Autodesk Inventor part; units mm, degrees
ref_plane "Work Plane1" through (-82.5, -59.605, 0) normal (0, 0, 1) x (1, 0, 0)
ref_plane "Work Plane2" through (-82.5, -59.605, 0) normal (0, 0, 1) x (1, 0, 0)
ref_plane "YZ Plane" through (0, 0, 0) normal (1, 0, 0) x (0, 1, 0)
ref_plane "Work Plane1" through (-82.5, -59.605, 0) normal (0, 0, 1) x (1, 0, 0)
sketch "Sketch1" plane through (0, 0, 0) normal (0, 0, 1) x (1, 0, 0)
  circle A0 centre (-78.95, -56.05) radius 1.75
  circle A1 centre (78.95, -56.05) radius 1.75
  circle A2 centre (78.95, 56.05) radius 1.75
  circle A3 centre (-78.95, 56.05) radius 1.75
  line L0 (-92.4724, 65.475) -> (91.6776, 65.475)
  line L1 (91.6776, 65.475) -> (91.6776, -64.7)
  line L2 (91.6776, -64.7) -> (-92.4724, -64.7)
  line L3 (-92.4724, -64.7) -> (-92.4724, 65.475)
  line L4 (-80.31, 46.61) -> (76.39, 46.61) construction
  line L5 (-80.31, -42.49) -> (-80.31, 46.61) construction
  line L6 (76.39, -42.49) -> (-80.31, -42.49) construction
  line L7 (76.39, 46.61) -> (76.39, -42.49) construction
  line L8 (-55.7212, -9.8482) -> (100.3438, -9.8482) construction
  line L9 (-82.2, -52) -> (82.2, -52) construction
  line L10 (-82.2, -52) -> (82.2, -52) construction
  circle A4 centre (-65.46, -58.76) radius 3.4
  circle A5 centre (-40.06, -58.76) radius 3.4
  circle A6 centre (-14.66, -58.76) radius 3.4
  circle A7 centre (10.74, -58.76) radius 3.4
  circle A8 centre (36.14, -58.76) radius 3.4
  circle A9 centre (61.54, -58.76) radius 3.4
  line L11 (82.5, -51.7) -> (82.5, 51.7)
  line L12 (82.2, 52) -> (-82.2, 52)
  line L13 (-82.5, 51.7) -> (-82.5, -51.7)
  line L14 (-82.2, -52) -> (82.2, -52)
  arc A10 (-82.2, 52) -> (-82.5, 51.7) centre (-82.2, 51.7) ccw
  arc A11 (82.5, 51.7) -> (82.2, 52) centre (82.2, 51.7) ccw
  arc A12 (82.2, -52) -> (82.5, -51.7) centre (82.2, -51.7) ccw
  arc A13 (-82.5, -51.7) -> (-82.2, -52) centre (-82.2, -51.7) ccw
  line L15 (-82.2, -53.27) -> (82.2, -53.27)
  arc A14 (82.2, -53.27) -> (83.77, -51.7) centre (82.2, -51.7) ccw
  line L16 (83.77, -51.7) -> (83.77, 51.7)
  arc A15 (83.77, 51.7) -> (82.2, 53.27) centre (82.2, 51.7) ccw
  line L17 (82.2, 53.27) -> (-82.2, 53.27)
  arc A16 (-82.2, 53.27) -> (-83.77, 51.7) centre (-82.2, 51.7) ccw
  line L18 (-83.77, 51.7) -> (-83.77, -51.7)
  arc A17 (-83.77, -51.7) -> (-82.2, -53.27) centre (-82.2, -51.7) ccw
  point P0 (-0.3974, -64.7)
  point P1 (-1.96, 65.475)
  dimension "d1" = 130.175
  dimension "d2" = 184.15
  dimension "d3" = 12.7
  dimension "d4" = 6.8
  dimension "d7" = 25.4
  dimension "d18" = 1.27
ref_plane "Work Plane2" through (-82.5, -59.605, 0) normal (0, 0, 1) x (1, 0, 0)
extrude "Extrusion2" add sketch "Sketch1" along normal blind 3.175 from surface at 0 contours L0 L1 L2 L3
properties part number "Center Bezel"
CAD build for the part. Positions are in the model's coordinates, mm. Coordinates: 2 decimals unless noted, no trailing zeros. Loops run counter-clockwise (first coordinate to the right, second up) from the corner with the lowest first, then second, coordinate; pieces in that order, holes last. Notation, with made-up numbers: (19.5, -24.75) - (59.5, -24.75) arc R16 ccw to (59.5, 1.25) - close; hole circle Ø11 at (34, 12.5). An arc over 180 degrees is marked (long way). Return JSON: item names as keys, results as strings.
1. Band-saw the part on B-B (x = -65.46). Give the cut face in (y, z) (3 decimals).
Result:
{"outline": "(-64.7, 0) - (-62.16, 0) - (-62.16, 3.175) - (-64.7, 3.175) - close; (-55.36, 0) - (-53.27, 0) - (-53.27, 3.175) - (-55.36, 3.175) - close; (53.27, 0) - (65.475, 0) - (65.475, 3.175) - (53.27, 3.175) - close"}
2. Drop a flat-ended pin along its axis: pin 1 (5.5 mm diameter, centred on x = 61.54, y = -58.76, fed in from +Z). Give the stop position or say it passes through.
Result:
{"pin 1": "passes through"}
3. Band-saw the part on A-A (y = -30.5). Give the cut face in (x, z) (3 decimals), and give its area (3 significant figures).
Result:
{"outline": "(-92.472, 0) - (-83.77, 0) - (-83.77, 3.175) - (-92.472, 3.175) - close; (83.77, 0) - (91.678, 0) - (91.678, 3.175) - (83.77, 3.175) - close", "area": "52.7 mm2"}
4. Band-saw the part on D-D (z = 1.9). State how many separate pieces and enclosed holes the cut face has, and give its area (3 significant figures).
Result:
{"separate pieces": "1", "enclosed holes": "11", "area": "5,870 mm2"}
5. Probe L1, parallel to Y at x = -40.06, z = 1.1 (3 decimals); L2, parallel to Y at x = 78.95, z = 1 (3 decimals); L3, parallel to X at y = -47, z = 1.25. List the from-to ranges inside material, lowest first. Write a range as from..to.
Result:
{"L1": "y = -64.7..-62.16, -55.36..-53.27, 53.27..65.475", "L2": "y = -64.7..-57.8, -54.3..-53.27, 53.27..54.3, 57.8..65.475", "L3": "x = -92.47..-83.77, 83.77..91.68"}
6. Band-saw the part on C-C (x = -20). Give the cut face in (y, z) (3 decimals).
Result:
{"outline": "(-64.7, 0) - (-53.27, 0) - (-53.27, 3.175) - (-64.7, 3.175) - close; (53.27, 0) - (65.475, 0) - (65.475, 3.175) - (53.27, 3.175) - close"}
7. Mould opens along X. For faces 1 (the cylindrical face through (64.7, -57.5, 1.6)), 2 (the flat face through (-1, 54, 0)) say: released by +X, released by -X, zero draft, split by the parting line, or undercut.
Result:
{"face 1": "undercut", "face 2": "zero draft"}
